Autodesk Inventor part; units mm, degrees
ref_plane "YZ Plane" through (0, 0, 0) normal (1, 0, 0) x (0, 1, 0)
ref_plane "XZ Plane" through (0, 0, 0) normal (0, 1, 0) x (-1, 0, 0)
ref_plane "XY Plane" through (0, 0, 0) normal (0, 0, 1) x (1, 0, 0)
sketch "Boceto1" plane through (0, 0, 0) normal (0, 1, 0) x (-1, 0, 0)
  line L0 (0, 0) -> (36, 0)
  line L1 (36, 0) -> (36, 0)
  line L2 (36, 0) -> (36, 77)
  line L3 (36, 77) -> (36, 77)
  line L4 (36, 77) -> (-36, 77)
  line L5 (-36, 77) -> (-36, 0)
  line L6 (-36, 0) -> (0, 0)
  line L7 (36, 77) -> (31, 77)
  line L8 (31, 77) -> (31, 72)
  line L9 (-36, 77) -> (-36, 77)
  line L10 (-36, 77) -> (-36, 72)
  line L11 (-36, 72) -> (-31, 72)
  circle A0 centre (-31, 72) radius 2
  circle A1 centre (31, 72) radius 2
  line L12 (36, 0) -> (0, 0)
  line L13 (0, 0) -> (0, 2.25)
  line L14 (0, 2.25) -> (2, 2.25)
  line L15 (2, 2.25) -> (2, 0)
  line L16 (0, 2.25) -> (-2, 2.25)
  line L17 (-2, 2.25) -> (-2, 0)
  line L18 (0, 0) -> (0, 50)
  line L19 (-12.5, 57) -> (12.5, 57)
  line L20 (12.5, 57) -> (12.5, 43)
  line L21 (12.5, 43) -> (-12.5, 43)
  line L22 (-12.5, 43) -> (-12.5, 57)
  line L23 (-12.5, 57) -> (12.5, 43) construction
  line L24 (12.5, 57) -> (-12.5, 43) construction
  line L25 (-12.5, 57) -> (12.5, 57)
  line L26 (12.5, 57) -> (12.5, 62.4)
  line L27 (12.5, 62.4) -> (-12.5, 62.4)
  line L28 (-12.5, 62.4) -> (-12.5, 57)
  line L29 (12.5, 62.4) -> (10, 62.4)
  line L30 (10, 62.4) -> (10, 59.9)
  line L31 (-12.5, 62.4) -> (-10, 62.4)
  line L32 (-10, 62.4) -> (-10, 59.9)
  circle A2 centre (10, 59.9) radius 1.75
  circle A3 centre (-10, 59.9) radius 1.75
  line L33 (-12.5, 62.4) -> (-12.5, 35.4)
  line L34 (-12.5, 35.4) -> (12.5, 35.4)
  line L35 (12.5, 35.4) -> (12.5, 62.4)
  line L36 (12.5, 62.4) -> (-12.5, 62.4)
  line L37 (-12.5, 35.4) -> (-10, 35.4)
  line L38 (-10, 35.4) -> (-10, 37.9)
  line L39 (12.5, 35.4) -> (12.5, 37.9)
  line L40 (12.5, 37.9) -> (10, 37.9)
  circle A4 centre (10, 37.9) radius 1.75
  circle A5 centre (-10, 37.9) radius 1.75
  circle A6 centre (31, 72) radius 4
  circle A7 centre (-31, 72) radius 4
  line L41 (0, 0) -> (0, 30)
  line L42 (0, 30) -> (0, 23)
  line L43 (0, 23) -> (7, 23)
  line L44 (7, 23) -> (7, 30)
  line L45 (7, 30) -> (-7, 30)
  line L46 (-7, 30) -> (-7, 23)
  line L47 (-7, 23) -> (0, 23)
  point P0 (2, 0)
  dimension "d0" = 36
  dimension "d1" = 0
  dimension "d2" = 77
  dimension "d3" = 0
  dimension "d4" = 72
  dimension "d5" = 5
  dimension "d6" = 5
  dimension "d7" = 0
  dimension "d8" = 5
  dimension "d9" = 5
  dimension "d10" = 4
  dimension "d11" = 4
  dimension "d14" = 36
  dimension "d15" = 2.25
  dimension "d16" = 2
  dimension "d17" = 2
  dimension "d18" = 50
  dimension "d19" = 25
  dimension "d20" = 14
  dimension "d21" = 5.4
  dimension "d22" = 2.5
  dimension "d23" = 2.5
  dimension "d24" = 2.5
  dimension "d25" = 2.5
  dimension "d26" = 3.5
  dimension "d27" = 3.5
  dimension "d28" = 27
  dimension "d29" = 25
  dimension "d30" = 2.5
  dimension "d31" = 2.5
  dimension "d32" = 2.5
  dimension "d33" = 2.5
  dimension "d34" = 3.5
  dimension "d35" = 3.5
  dimension "d50" = 8
  dimension "d51" = 8
  dimension "d61" = 30
  dimension "d63" = 7
  dimension "d64" = 14
  dimension "d65" = 7
  dimension "d66" = 0
extrude "Extrusión1" add sketch "Boceto1" against normal blind 3 contours A6 | A7 | A5 | L34 L33 L21 L18 | A4 | L18 L21 L35 L34 | L15 L14 L16 L17 L6 L5 L4 L2 L0 | A2 | A3 | L19 L28 L27 L26
extrude "Extrusión2" cut sketch "Boceto1" against normal blind 1.5 contours A5 | A4 | A2 | A3
thread "Rosca1"
thread "Rosca2"
thread "Rosca3"
thread "Rosca4"
thread "Rosca5"
thread "Rosca6"
extrude "Extrusión3" [suppressed]
equation "\"d0\" = 0.5 * box_in_width"
equation "\"d2\" = box_in_deep"
equation "\"d4\" = box_in_width"
equation "\"d5\" = offset + 0.5 * screw_Dhead"
equation "\"d6\" = offset + 0.5 * screw_Dhead"
equation "\"d8\" = offset + 0.5 * screw_Dhead"
equation "\"d9\" = offset + 0.5 * screw_Dhead"
equation "\"d10\" = screw_d"
equation "\"d11\" = screw_d"
equation "\"d14\" = 0.5 * box_in_width"
equation "\"d15\" = 1.5 * thikness_box"
equation "\"d19\" = screen_width"
equation "\"d20\" = screen_height"
equation "\"d21\" = top_from_screen"
equation "\"d22\" = offset_screw_screen + 0.5 * screw_d_screen"
equation "\"d23\" = offset_screw_screen + 0.5 * screw_d_screen"
equation "\"d24\" = offset_screw_screen + 0.5 * screw_d_screen"
equation "\"d25\" = offset_screw_screen + 0.5 * screw_d_screen"
equation "\"d28\" = height_screen_total"
equation "\"d29\" = screen_width"
equation "\"d30\" = offset_screw_screen + 0.5 * screw_d_screen"
equation "\"d31\" = offset_screw_screen + 0.5 * screw_d_screen"
equation "\"d32\" = offset_screw_screen + 0.5 * screw_d_screen"
equation "\"d33\" = offset_screw_screen + 0.5 * screw_d_screen"
equation "\"d50\" = screw_Dhead"
equation "\"d51\" = screw_Dhead"
equation "\"d64\" = 2 * d63"
equation "\"d12\" = 2 * thikness_box"
equation "\"d36\" = deep_screw_screen"
equation "\"thikness\" = 2"
equation "\"offset\" = 1"
equation "\"r1\" = 5.55"
equation "\"r2o\" = 59.75"
equation "\"delta_y\" = 6"
equation "\"wire_d\" = 1"
equation "\"width_ang_spring\" = 5"
equation "\"spring_int_diam\" = 8.5"
equation "\"spring_ext_diam\" = 10.5"
equation "\"r3\" = 8.25"
equation "\"r3R\" = 4.75"
equation "\"r3T\" = 6.74537"
equation "\"alpha\" = 54.847297deg"
equation "\"alpha2\" = 270deg"
equation "\"theta3_recogido\" = 305.152703deg"
equation "\"delta_theta_3\" = 45deg"
equation "\"joint_width\" = 12"
equation "\"joint_radius\" = 7.75"
equation "\"shaft_width\" = 15"
equation "\"shaft_joint_diameter\" = 7.75"
equation "\"separation_space\" = 0.5"
equation "\"height_finger\" = 42"
equation "\"cell_screw_head_diameter\" = 4"
equation "\"cell_screw_diameter\" = 2"
equation "\"cell_space\" = 2"
equation "\"cell_width\" = 6"
equation "\"cell_theta_position\" = 60deg"
equation "\"cell_thikness\" = 1"
equation "\"cell_lenght\" = 37"
equation "\"cell_z_space\" = 5"
equation "\"wire_D\" = 2.3"
equation "\"width_link\" = 8"
equation "\"Dt\" = 1.05949"
equation "\"Djoint_shaft\" = 2.3"
equation "\"shaft_x\" = 1.45"
equation "\"shaft_y\" = 6.45"
equation "\"lenght_body_link\" = 186.05"
equation "\"lenght_bar_support\" = 201.65"
equation "\"wire_spring_d\" = 1"
equation "\"spring_int_d\" = 6"
equation "\"spring_lenght\" = 28"
equation "\"trigger_offset\" = 2"
equation "\"m2_theta2o\" = 107deg"
equation "\"m2_r2\" = 28"
equation "\"e\" = 9"
equation "\"So\" = 17"
equation "\"m2_theta3o\" = -30deg"
equation "\"m2_r3\" = 19.75"
equation "\"m2_delta_theta1\" = 15deg"
equation "\"m2_theta3f\" = -60deg"
equation "\"trigger_thumb_lenght\" = 6"
equation "\"width_r12\" = 8"
equation "\"m2_r1\" = 25.2"
equation "\"r3_thikness\" = 3.5"
equation "\"t_thikness\" = 3"
equation "\"tg_width\" = 4"
equation "\"pivot_screw_d\" = 4"
equation "\"pivot_diameter\" = 7"
equation "\"sj_diam_shaft\" = 6"
equation "\"sj_groove\" = 2"
equation "\"sj_groove_deep\" = 7"
equation "\"sj_head_D\" = 7"
equation "\"sj_head_d\" = 4.7464"
equation "\"sj_head_height\" = 5"
equation "\"sf_lenght\" = 9.5"
equation "\"sf_base\" = 3"
equation "\"sf_head_height\" = 3"
equation "\"sf_head_width\" = 4.5"
equation "\"sf_head_offset\" = 0.25"
equation "\"sf_head_grip_width\" = 2"
equation "\"sf_head_angle\" = 45deg"
equation "\"sf_thikness\" = 5"
equation "\"screw_Dhead\" = 8"
equation "\"screw_d\" = 4"
equation "\"screw_lenght\" = 12"
equation "\"screwJ_base_D\" = 9"
equation "\"screwJ_top_D\" = 13"
equation "\"gj_D\" = 6"
equation "\"gj_d\" = 4"
equation "\"gj_out_section\" = 6"
equation "\"box_in_deep\" = 77"
equation "\"box_in_width\" = 72"
equation "\"box_in_height\" = 35"
equation "\"thikness_box\" = 1.5"
equation "\"box_slim_slider_lenght\" = 116"
equation "\"sf_flex_separation\" = 38.66667"
equation "\"flex_separation_theta\" = 60deg"
equation "\"box_fat_slider_lenght\" = 67"
equation "\"int_width_slider\" = 2"
equation "\"ext_width_slider\" = 3.5"
equation "\"fat_width_slider\" = 2"
equation "\"slim_width_slider\" = 1.5"
equation "\"sfbox_width\" = 1.5"
equation "\"sfbox_tip_width\" = 2.5"
equation "\"sfbox_theta1\" = 60deg"
equation "\"sfbox_theta2\" = 45deg"
equation "\"agarradera_theta\" = 60deg"
equation "\"agarradera_width\" = 4"
equation "\"agarradera_position\" = 82.13077"
equation "\"screen_width\" = 25"
equation "\"screen_height\" = 14"
equation "\"screw_d_screen\" = 3"
equation "\"offset_screw_screen\" = 1"
equation "\"height_screen_total\" = 27"
equation "\"top_from_screen\" = 5.4"
equation "\"deep_screw_screen\" = 1.5"
properties part number "Box_cover"
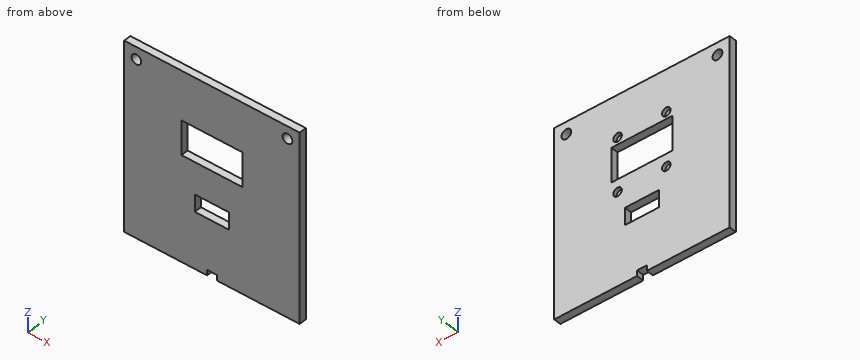
Read the model definition and answer for the solid it produces. Units are mm, in the model's axes. Coordinates: 2 decimals unless noted, no trailing zeros. Order: outer loops, then holes, each group sorted by start corner. A loop starts at its lowest first (then second) coordinate and runs counter-clockwise, first axis right, second up. Notation, with made-up numbers: M 20,30 L 57,30 A34 cw 57,60 Z; hole C 11,-28.75 d5. An arc over 180 degrees is marked long. Put each result on its own line as item: value. Start each with the question number.
Item 1: Given pin 1 Ø1 at (x, z) = (-9.5, 38) entering from +Y; pin 2 Ø0.9 at (x, y) = (0.5, -1.5) entering from -Z, each flat-ended and moving along its own axis, determine where each tip first touches the part or whether it passes through.
Item 2: Section D-D, the plane z = 72 is taken. Determine the outline of the cut face in (x, y), plus the area to 3 significant figures.
Item 3: Consider probe 1 along X at (y, z) = (-1.15, 72); probe 2 along Z at (x, y) = (6, -1.3); probe 3 along X at (y, z) = (-2.5, 29.5). Determine where each line is inside the solid, lowest interval first. Write a range as [from, to].
Item 4: Section A-A, the plane x = -10 is taken. Determine the outline of the cut face in (y, z).
Item 5: Section C-C, the plane x = 4 is taken. Determine the outline of the cut face in (y, z), plus the area to 3 significant figures.
Item 6: Section B-B, the plane z = 48 is taken. Determine the outline of the cut face in (x, y).
Computed:
1. pin 1: stops at y = -1.5
1. pin 2: stops at z = 2.25
2. outline: M -36,-3 L -33,-3 L -33,0 L -36,0 Z; M -29,-3 L 29,-3 L 29,0 L -29,0 Z; M 33,-3 L 36,-3 L 36,0 L 33,0 Z
2. area: 192 mm2
3. probe 1: x = [-36, -33], [-29, 29], [33, 36]
3. probe 2: z = [0, 23], [30, 43], [57, 77]
3. probe 3: x = [-36, -7], [7, 36]
4. outline: M -3,0 L 0,0 L 0,36.15 L -1.5,36.15 L -1.5,39.65 L 0,39.65 L 0,43 L -3,43 Z; M -3,57 L 0,57 L 0,58.15 L -1.5,58.15 L -1.5,61.65 L 0,61.65 L 0,77 L -3,77 Z
5. outline: M -3,0 L 0,0 L 0,23 L -3,23 Z; M -3,30 L 0,30 L 0,43 L -3,43 Z; M -3,57 L 0,57 L 0,77 L -3,77 Z
5. area: 168 mm2
6. outline: M -36,-3 L -12.5,-3 L -12.5,0 L -36,0 Z; M 12.5,-3 L 36,-3 L 36,0 L 12.5,0 Z
